Can you work these out from the model? Positions are in its coordinate system, mm. A direction names the side the tool comes from. Give positions to 0.01 mm unless a question says otherwise; leave off trailing zeros. Loops run counter-clockwise (first coordinate to the right, second up) from the corner with the lowest first, then second, coordinate; pieces in that order, holes last. Notation, with made-up numbers: (78.5, 27) - (113.5, 27) arc R9 ccw to (113.5, 43) - close; hole circle Ø1 at (-29.5, 54.25). An arc over 180 degrees is marked (long way). Answer as a JSON object with one key per item and string values.
```python
from build123d import *

# Parameters (mm, degrees)
SKETCH_1_W            = 330
SKETCH_1_H            = 33.5
EXTRUDE_1_DEPTH       = 8.5
SKETCH_2_W            = 23.5
SKETCH_2_H            = 5.5
CUT_EXTRUDE_1_DEPTH   = 332.804912562
HOLE_WIZARD_5_0_5_1_D = 5


with BuildPart() as part:
    # Эскиз1 → Бобышка-Вытянуть1 (new body)
    with BuildSketch(Plane(origin=(0, 8.5, 0), x_dir=(1, 0, 0), z_dir=(0, 1, 0))):
        with Locations((165, -16.75)):
            Rectangle(SKETCH_1_W, SKETCH_1_H)
    extrude(amount=-EXTRUDE_1_DEPTH)

    # Эскиз2 → Вырез-Вытянуть1 (cut, through all)
    with BuildSketch(Plane(origin=(330, 0, 0), x_dir=(0, 0, -1), z_dir=(1, 0, 0))):
        with Locations((-16.75, 5.75)):
            Rectangle(SKETCH_2_W, SKETCH_2_H)
    extrude(amount=-CUT_EXTRUDE_1_DEPTH, mode=Mode.SUBTRACT)

    # Диаметр отверстия Ø5.0 (5)1 (through all)
    with Locations(Plane(origin=(0, 3, 0), x_dir=(1, 0, 0), z_dir=(0, 1, 0))):
        with Locations((65, -16.75), (125, -16.75), (265, -16.75), (205, -16.75)):
            Hole(HOLE_WIZARD_5_0_5_1_D / 2)


solid = part.part
```
1) Imagine slicing it at B-B on x = 31.5. Write out the boundary of the cut face in (y, z), and give its area (4 significant figures).
Check sheet entries:
{"outline": "(0, 0) - (8.5, 0) - (8.5, 5) - (3, 5) - (3, 28.5) - (8.5, 28.5) - (8.5, 33.5) - (0, 33.5) - close", "area": "155.5 mm2"}
2) If we mould it in two halves opening along Z, with no side actions, what happens to faces 1 (the flat face through (0, 2, 17)), 2 (the flat face through (163, 4, 33.5)), 3 (the cylindrical face through (202.69, 1.48, 17.71)), 4 (the flat face through (167, 6, 28.5))? For each: released by +Z, released by -Z, zero draft, split by the parting line, or undercut.
Check sheet entries:
{"face 1": "zero draft", "face 2": "released by +Z", "face 3": "undercut", "face 4": "undercut"}
3) I need wall thicknesses on L1, parallel to X at y = 1.1, z = 16.75; L2, parallel to Z at x = 309.5, y = 3.75; L3, parallel to Z at x = 265, y = 0.8. Which ranges of each line are inside material? Lowest first, please.
Check sheet entries:
{"L1": "0 to 62.5, 67.5 to 122.5, 127.5 to 202.5, 207.5 to 262.5, 267.5 to 330", "L2": "0 to 5, 28.5 to 33.5", "L3": "0 to 14.25, 19.25 to 33.5"}
4) Which directions (+Z, -Z, +X, -X, +Y, -Y) give clear straight access to the entire face, cutting with the end or side of a thin tool? Please do faces 5 (the flat face through (163, 8.5, 2)), 6 (the flat face through (167, 6, 5)).
Check sheet entries:
{"face 5": "+Z, -Z, +X, -X, +Y", "face 6": "+X, -X, +Y"}
5) Imagine slicing it at A-A on y = 6.5. Write out the boundary of the cut face in (x, z), and give its area (3 significant figures).
Check sheet entries:
{"outline": "(0, 0) - (330, 0) - (330, 5) - (0, 5) - close; (0, 28.5) - (330, 28.5) - (330, 33.5) - (0, 33.5) - close", "area": "3,300 mm2"}
6) I'm going to push a flat-ended pin straight in: P1, Ø12, axis at x = 140, z = 14, coming from the +Y side. Where does the tip first touch, or does it pass through?
Check sheet entries:
{"P1": "y = 3"}
